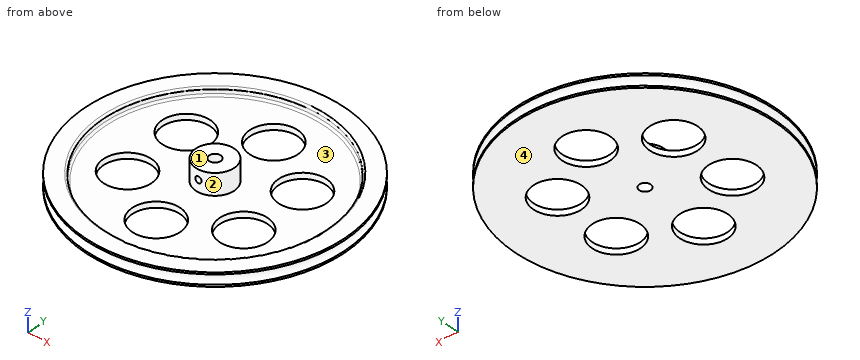
```python
from build123d import *

# Parameters (mm, degrees)
CYLINDER002_R     = 10
CYLINDER002_DEPTH = 14
CYLINDER001_R     = 58
CYLINDER001_DEPTH = 4
CYLINDER_R        = 67.5
CYLINDER_DEPTH    = 7
SKETCH_R          = 3
HOLE_DEPTH        = 14.001
SKETCH001_R       = 2.5
SKETCH002_R       = 12.5
HOLE001_DEPTH     = 3.001
SKETCH003_R       = 1.65
HOLE002_DEPTH     = 9.00858
HOLE002_TIPS_R    = 1.65
FILLET_R          = 1
FILLET001_R       = 1


with BuildPart() as zylinder002:
    # Cylinder002 → Cylinder002 (new body)
    with BuildSketch(Plane.XY):
        Circle(CYLINDER002_R)
    extrude(amount=CYLINDER002_DEPTH)


with BuildPart() as zylinder001:
    # Cylinder001 → Cylinder001 (new body)
    with BuildSketch(Plane.XY.offset(3)):
        Circle(CYLINDER001_R)
    extrude(amount=CYLINDER001_DEPTH)


with BuildPart() as body:
    # Cylinder → Cylinder (new body)
    with BuildSketch(Plane.XY):
        Circle(CYLINDER_R)
    extrude(amount=CYLINDER_DEPTH)

    # Cut: cut Zylinder001
    add(zylinder001.part, mode=Mode.SUBTRACT)

    # Fusion: union Zylinder002
    add(zylinder002.part)

    # Sketch (on Face1 of BaseFeature) → Hole (cut, through all)
    with BuildSketch(Plane.XY.offset(14)):
        Circle(SKETCH_R)
    extrude(amount=-HOLE_DEPTH, mode=Mode.SUBTRACT)

    # Sketch001 → Groove (revolve, cut)
    with BuildSketch(Plane.YZ):
        with Locations((67.5, 3.5)):
            Circle(SKETCH001_R)
    revolve(axis=Axis((0, 0, 0), (0, 0, 1)), mode=Mode.SUBTRACT)

    # Sketch002 (on Face4 of Groove) → Hole001 (cut, through all)
    with BuildSketch(Plane.XY.offset(3)):
        with Locations((0, 35)):
            Circle(SKETCH002_R)
        with Locations((30.310889, 17.5)):
            Circle(SKETCH002_R)
        with Locations((30.310889, -17.5)):
            Circle(SKETCH002_R)
        with Locations((-30.310889, -17.5)):
            Circle(SKETCH002_R)
        with Locations((0, -35)):
            Circle(SKETCH002_R)
        with Locations((-30.310889, 17.5)):
            Circle(SKETCH002_R)
    extrude(amount=-HOLE001_DEPTH, mode=Mode.SUBTRACT)

    # Sketch003 → Hole002 (cut)
    with BuildSketch(Plane.XZ.offset(10)):
        with Locations((0, 9)):
            Circle(SKETCH003_R)
    extrude(amount=-HOLE002_DEPTH, mode=Mode.SUBTRACT)

    # Hole002 tips → Hole002 tip 1 section 0
    with BuildSketch(Plane.XZ.offset(0.99142), mode=Mode.PRIVATE) as hole002_tip_1_s0:
        with Locations((0, 9)):
            Circle(HOLE002_TIPS_R)
    loft([hole002_tip_1_s0.sketch, Vertex(0, 0, 9)], mode=Mode.SUBTRACT)

    # Fillet
    fillet_edges = [body.edges().sort_by_distance(p)[0] for p in [
        (-58, 0, 7),
    ]]
    fillet(fillet_edges, radius=FILLET_R)

    # Fillet001
    fillet001_edges = [body.edges().sort_by_distance(p)[0] for p in [
        (-58, 0, 3),
    ]]
    fillet(fillet001_edges, radius=FILLET001_R)


solid = body.part
```
The listing builds one solid part. Answer for the finished solid, in the listing's coordinates (mm). Face numbers are marked on the shaded views. A direction names the side the tool comes from. Round coordinates to 2 decimals unless told otherwise and drop trailing zeros.
1) Consider line 1 (Y direction, x = 0, z = 2); line 2 (Y direction, x = 0, z = 5.6); line 3 (Z direction, x = 0, y = -5.25). Determine where each line is inside the solid, lowest interval first.
Outcome:
line 1: y = -65.5 to -47.5, -22.5 to -3, 3 to 22.5, 47.5 to 65.5
line 2: y = -66.14 to -58, -10 to -3, 3 to 10, 58 to 66.14
line 3: z = 0 to 7.35, 10.65 to 14
2) Given P1, Ø3.5, axis at x = 0, y = 0, coming from the +Z side; P2, Ø6, axis at x = -21.5, z = 2.5, coming from the -Y side; P3, Ø6, axis at y = -42.5, z = 7, coming from the +X side; P4, Ø8, axis at y = -36.5, z = 8.5, coming from the -X side, each flat-ended and moving along its own axis, determine where each tip first touches the part or whether it passes through.
Outcome:
P1: passes through
P2: stops at y = -64.8
P3: stops at x = 54.74
P4: stops at x = -59
3) For the marked faces 1 and 2, determine the directions among +Z, -Z, +X, -X, +Y, -Y from which every point of the face is accessible in a straight line to the end or side of a thin tool.
Outcome:
face 1: +Z, +X, -X, +Y, -Y
face 2: +Z
4) For a pull along X with two mould halves and no side action, classify the marked faces 3 and 4 as released by +X, released by -X, zero draft, split by the parting line, or undercut.
Outcome:
face 3: undercut
face 4: zero draft
5) A cutting plane is placed at A-A on x = -26.5. Give the number of separate pieces and of enclosed holes in the cut face, plus the area to 3 significant figures.
Outcome:
separate pieces: 3
enclosed holes: 0
area: 292 mm2
